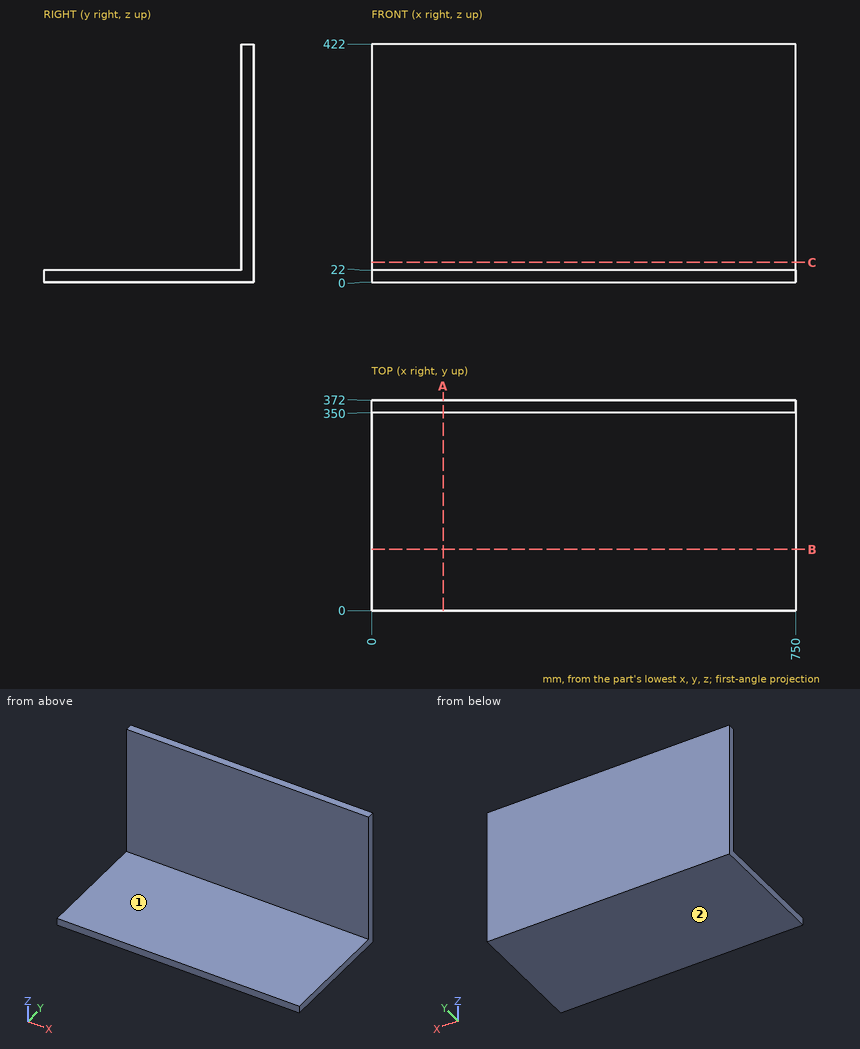
Job drawing, mm, ordinate dimensions from the low corner. One solid piece. A direction names the side the tool comes from. Round coordinates to 2 decimals unless told otherwise and drop trailing zeros. Order: outer loops, then holes, each group sorted by start corner. A loop starts at its lowest first (then second) coordinate and runs counter-clockwise, first axis right, second up. Notation, with made-up numbers: M -10.5,-2.75 L 30.5,-2.75 A24 cw 30.5,32.25 Z; hole C -21.75,24 d6. An arc over 180 degrees is marked long. Write each question's results on one line, items separated by ' | '. Start each with the question number.
(1) Probe probe 1 along Z at (x, y) = (457, 21); probe 2 along Y at (x, z) = (158.5, 245.5). List the from-to ranges inside material, lowest first. Write a range as from..to.
(2) Drop flat-ended pins along their axis: pin 1 (2 mm diameter, centred on x = 668.5, z = 183.5, fed in from -Y); pin 2 (8 mm diameter, centred on x = 476, y = 192, fed in from +Z). Give the stop position or say it passes through.
(3) Saw through at A-A, the plane x = 126.5. Give the cut face in (y, z).
(4) Saw through at B-B, the plane y = 108.5. Give the cut face in (x, z), then the cut area to 3 significant figures.
(5) Saw through at C-C, the plane z = 35.5. Give the cut face in (x, y), then the cut area to 3 significant figures.
(6) Which spindle directions (+Z, -Z, +X, -X, +Y, -Y) get a long thin tool onto all of the face, cutting with end or side? Do the marked faces 1 and 2. Say none if no direction does.
Established:
1) probe 1: z = 0..22 | probe 2: y = 350..372
2) pin 1: stops at y = 350 | pin 2: stops at z = 22
3) outline: M 0,0 L 372,0 L 372,422 L 350,422 L 350,22 L 0,22 Z
4) outline: M 0,0 L 750,0 L 750,22 L 0,22 Z | area: 16,500 mm^2
5) outline: M 0,350 L 750,350 L 750,372 L 0,372 Z | area: 16,500 mm^2
6) face 1: +Z, +X, -X, -Y | face 2: -Z, +X, -X, +Y, -Y
